```python
from build123d import *

# Parameters (mm, degrees)
SKETCH020_W     = 31.6
SKETCH020_H     = 31.6
PAD010_DEPTH    = 4
CHAMFER_SIZE    = 3
FILLET011_R     = 2
SKETCH021_W     = 5.6
SKETCH021_H     = 5.6
PAD011_DEPTH    = 6.7
SKETCH022_R     = 2
POCKET004_DEPTH = 6.7


with BuildPart() as part:
    # Sketch020 → Pad010 (new body)
    with BuildSketch(Plane.XY):
        Rectangle(SKETCH020_W, SKETCH020_H)
        Polygon((0, 8), (-5.656854, 5.656854), (-8, 0), (-5.656854, -5.656854), (0, -8), (5.656854, -5.656854), (8, 0), (5.656854, 5.656854), align=None, mode=Mode.SUBTRACT)
    extrude(amount=-PAD010_DEPTH)

    # Chamfer
    chamfer_edges = [part.edges().sort_by_distance(p)[0] for p in [
        (2.828427, 6.828427, 0),
        (6.828427, 2.828427, 0),
        (6.828427, -2.828427, 0),
        (2.828427, -6.828427, 0),
        (-2.828427, -6.828427, 0),
        (-6.828427, -2.828427, 0),
        (-6.828427, 2.828427, 0),
        (-2.828427, 6.828427, 0),
    ]]
    chamfer(chamfer_edges, length=CHAMFER_SIZE)

    # Fillet011
    fillet011_edges = [part.edges().sort_by_distance(p)[0] for p in [
        (-6.804905, 6.804905, -1.5),
        (0, 9.623588, -1.5),
        (6.804905, 6.804905, -1.5),
        (9.623588, 0, -1.5),
        (-6.804905, -6.804905, -1.5),
        (-9.623588, 0, -1.5),
        (0, -9.623588, -1.5),
        (6.804905, -6.804905, -1.5),
    ]]
    fillet(fillet011_edges, radius=FILLET011_R)

    # Sketch021 (on Face4 of Fillet011) → Pad011 (join)
    with BuildSketch(Plane(origin=(0, 0, -4), x_dir=(1, 0, 0), z_dir=(0, 0, -1))):
        with Locations((-13, -13)):
            Rectangle(SKETCH021_W, SKETCH021_H)
        with Locations((13, -13)):
            Rectangle(SKETCH021_W, SKETCH021_H)
        with Locations((13, 13)):
            Rectangle(SKETCH021_W, SKETCH021_H)
        with Locations((-13, 13)):
            Rectangle(SKETCH021_W, SKETCH021_H)
    extrude(amount=PAD011_DEPTH)

    # Sketch022 (on Face43 of Pad011) → Pocket004 (cut)
    with BuildSketch(Plane(origin=(0, 0, -10.7), x_dir=(1, 0, 0), z_dir=(0, 0, -1))):
        with Locations((-13, 13)):
            Circle(SKETCH022_R)
        with Locations((13, 13)):
            Circle(SKETCH022_R)
        with Locations((13, -13)):
            Circle(SKETCH022_R)
        with Locations((-13, -13)):
            Circle(SKETCH022_R)
    extrude(amount=-POCKET004_DEPTH, mode=Mode.SUBTRACT)


solid = part.part
```
Can you work these out from the model? Positions are in its coordinate system, mm. A direction names the side the tool comes from. Coordinates: 2 decimals unless noted, no trailing zeros. Write each loop counter-clockwise with the first axis right and the second up, starting at its lowest first coordinate (ties: lowest second). Pieces come first, ordered by that corner, then holes. Notation, with made-up numbers: M 15.5,65.5 L 21.5,65.5 A27 cw 21.5,101.5 Z; hole C -24.75,11.25 d7. An arc over 180 degrees is marked long. Write item = value, one per line. Start each with the question number.
Q1. If we section it at D-D, the plane x = -1: Write out the boundary of the cut face in (y, z), then the cut area to 3 significant figures.
Q2. I'm going to push a flat-ended pin straight in: pin 1 (8 mm diameter, centred on x = -4, y = -3, fed in from -Z). Where does the tip first touch, or does it pass through?
Q3. If we section it at B-B, the plane x = -13: Write out the boundary of the cut face in (y, z).
Q4. Thinking about a two-plate mould opening in Y: for faces 4 (the face through (10.2, -13, -7)), 5 (the face through (-6.73, -6.72, -1.5)), which applies, released by +Y, released by -Y, zero draft, split by the parting line, or undercut?
Q5. If we section it at A-A, the plane z = -6.5: Write out the boundary of the cut face in (x, y).
Q6. On a 3-axis mill with a long thin cutter (end or side, diameter ignored), from which of +Z, -Z, +X, -X, +Y, -Y can I reach the whole of each face in a straight line? I mean faces 1 (the face through (-3.46, -8.21, -1.48)), 2 (the face through (-13, 13, -4)), 3 (the face through (-6.845, -2.789, -3.562)). Say none if no direction works.
Q7. If I drill on L1, parallel to Y at x = 13, z = -6.75; L2, parallel to X at y = -12.5, z = -6.75, over which ranges is the centre line in solid material (lowest first)? Write a range as [from, to].
Q8. If we section it at C-C, the plane y = -2: Write out the boundary of the cut face in (x, z), then the cut area to 3 significant figures.
Check sheet entries:
q1.outline = M -15.8,-4 L -7.59,-4 L -7.59,-3 L -10.83,0 L -15.8,0 Z; M 7.59,-4 L 15.8,-4 L 15.8,0 L 10.83,0 L 7.59,-3 Z
q1.area = 56.0 mm²
q2.pin_1 = -4
q3.outline = M -15.8,-10.7 L -15,-10.7 L -15,-4 L -11,-4 L -11,-10.7 L -10.2,-10.7 L -10.2,-4 L 10.2,-4 L 10.2,-10.7 L 11,-10.7 L 11,-4 L 15,-4 L 15,-10.7 L 15.8,-10.7 L 15.8,0 L -15.8,0 Z
q4.face_4 = zero draft
q4.face_5 = undercut
q5.outline = M -15.8,-15.8 L -10.2,-15.8 L -10.2,-10.2 L -15.8,-10.2 Z; M -15.8,10.2 L -10.2,10.2 L -10.2,15.8 L -15.8,15.8 Z; M 10.2,-15.8 L 15.8,-15.8 L 15.8,-10.2 L 10.2,-10.2 Z; M 10.2,10.2 L 15.8,10.2 L 15.8,15.8 L 10.2,15.8 Z; hole C -13,-13 d4; hole C -13,13 d4; hole C 13,-13 d4; hole C 13,13 d4
q6.face_1 = +Z
q6.face_2 = -Z
q6.face_3 = +Z, -Z
q7.L1 = [-15.8, -15], [-11, -10.2], [10.2, 11], [15, 15.8]
q7.L2 = [-15.8, -14.94], [-11.06, -10.2], [10.2, 11.06], [14.94, 15.8]
q8.outline = M -15.8,-4 L -7.17,-4 L -7.17,-3 L -10.42,0 L -15.8,0 Z; M 7.17,-4 L 15.8,-4 L 15.8,0 L 10.42,0 L 7.17,-3 Z
q8.area = 59.3 mm²
